```python
from build123d import *

# Parameters (mm, degrees)
SKETCH1_W           = 27.94
SKETCH1_H           = 391.16
BOSS_EXTRUDE1_DEPTH = 3.81
SKETCH2_R           = 10
CUT_EXTRUDE1_DEPTH  = 3.21
BOSS_EXTRUDE2_DEPTH = 3.81
SKETCH5_W           = 46.80460671
SKETCH5_H           = 4.064
CUT_EXTRUDE2_DEPTH  = 182.88
BOSS_EXTRUDE3_DEPTH = 3.81


with BuildPart() as part:
    # Sketch1 → Boss-Extrude1 (new body)
    with BuildSketch(Plane(origin=(0, 0, 0), x_dir=(1, 0, 0), z_dir=(0, 1, 0))):
        Rectangle(SKETCH1_W, SKETCH1_H)
    extrude(amount=BOSS_EXTRUDE1_DEPTH)

    # Sketch2 → Cut-Extrude1 (cut)
    with BuildSketch(Plane(origin=(0, 3.81, 0), x_dir=(1, 0, 0), z_dir=(0, 1, 0))):
        with Locations(Location((0, 177.8, 0), (0, 0, 270))):
            Circle(SKETCH2_R)
        with Locations(Location((0, 152.4, 0), (0, 0, 270))):
            Circle(SKETCH2_R)
        with Locations(Location((0, 127, 0), (0, 0, 270))):
            Circle(SKETCH2_R)
        with Locations(Location((0, 101.6, 0), (0, 0, 270))):
            Circle(SKETCH2_R)
        with Locations(Location((0, 76.2, 0), (0, 0, 270))):
            Circle(SKETCH2_R)
        with Locations(Location((0, 50.8, 0), (0, 0, 270))):
            Circle(SKETCH2_R)
        with Locations(Location((0, 25.4, 0), (0, 0, 270))):
            Circle(SKETCH2_R)
        with Locations(Location((0, 0, 0), (0, 0, 270))):
            Circle(SKETCH2_R)
        with Locations(Location((0, -25.4, 0), (0, 0, 270))):
            Circle(SKETCH2_R)
        with Locations(Location((0, -50.8, 0), (0, 0, 270))):
            Circle(SKETCH2_R)
        with Locations(Location((0, -76.2, 0), (0, 0, 270))):
            Circle(SKETCH2_R)
        with Locations(Location((0, -101.6, 0), (0, 0, 270))):
            Circle(SKETCH2_R)
        with Locations(Location((0, -127, 0), (0, 0, 270))):
            Circle(SKETCH2_R)
        with Locations(Location((0, -152.4, 0), (0, 0, 270))):
            Circle(SKETCH2_R)
        with Locations(Location((0, -177.8, 0), (0, 0, 270))):
            Circle(SKETCH2_R)
    extrude(amount=-CUT_EXTRUDE1_DEPTH, mode=Mode.SUBTRACT)

    # Sketch4 → Boss-Extrude2 (add)
    with BuildSketch(Plane(origin=(0, 0, 0), x_dir=(1, 0, 0), z_dir=(0, 1, 0))):
        Polygon((23.402303355, -54.881033493), (13.97, -56.20665728), (13.97, -72.402209707), (23.402303355, -73.727833493), align=None)
        Polygon((23.402303355, 146.105623787), (13.97, 144.78), (13.97, 128.584447573), (23.402303355, 127.258823787), align=None)
        Polygon((-13.97, 128.584447573), (-13.97, 144.78), (-23.402303355, 146.105623787), (-23.402303355, 127.258823787), align=None)
        Polygon((23.402303355, 79.11007136), (13.97, 77.784447573), (13.97, 61.588895147), (23.402303355, 60.26327136), align=None)
        Polygon((23.402303355, 12.114518933), (13.97, 10.788895147), (13.97, -5.40665728), (23.402303355, -6.732281067), align=None)
        Polygon((-13.97, -5.40665728), (-13.97, 10.788895147), (-23.402303355, 12.114518933), (-23.402303355, -6.732281067), align=None)
        Polygon((-13.97, 61.588895147), (-13.97, 77.784447573), (-23.402303355, 79.11007136), (-23.402303355, 60.26327136), align=None)
        Polygon((23.402303355, -121.87658592), (13.97, -123.202209707), (13.97, -139.397762134), (23.402303355, -140.72338592), align=None)
        Polygon((-13.97, -139.397762134), (-13.97, -123.202209707), (-23.402303355, -121.87658592), (-23.402303355, -140.72338592), align=None)
        Polygon((-13.97, -72.402209707), (-13.97, -56.20665728), (-23.402303355, -54.881033493), (-23.402303355, -73.727833493), align=None)
    extrude(amount=BOSS_EXTRUDE2_DEPTH)

    # Sketch5 → Cut-Extrude2 (cut)
    with BuildSketch(Plane.XY.offset(195.58)):
        with Locations((0, 2.032)):
            Rectangle(SKETCH5_W, SKETCH5_H)
    extrude(amount=-CUT_EXTRUDE2_DEPTH, mode=Mode.SUBTRACT)

    # Sketch6 → Boss-Extrude3 (add)
    with BuildSketch(Plane(origin=(0, 3.81, 0), x_dir=(1, 0, 0), z_dir=(0, 1, 0))):
        Polygon((-4.80197372, -12.7), (-4.445, -15.24), (-13.97, -15.24), (-13.97, -12.7), align=None)
        Polygon((13.97, -12.7), (13.97, -15.24), (4.445, -15.24), (4.80197372, -12.7), align=None)
    extrude(amount=-BOSS_EXTRUDE3_DEPTH)


solid = part.part
```
Could you check a few things on this model? Use its own coordinates, in mm. A direction names the side the tool comes from. Give positions to 0.01 mm unless a question says otherwise; leave off trailing zeros. Loops run counter-clockwise (first coordinate to the right, second up) from the corner with the lowest first, then second, coordinate; pieces in that order, holes last. Notation, with made-up numbers: (52.5, 58) - (79.5, 58) arc R9 cw to (79.5, 62) - close; hole circle Ø8 at (37.25, 61). An arc over 180 degrees is marked (long way). Answer in a Markdown table with one row per item. Add a question column.
Q1. If we section it at C-C (y = 1.45): State how many separate pieces and enclosed holes the cut face has, plus the area to 3 significant figures.
Q2. We'd pull the mould along Z, two halves only. Please class faces 4 (the face through (13.97, 2, 10)), 5 (the face through (-18.752, 1.878, -127.912)), 6 (the face through (18.62, 1.878, -60.935)), 7 (the face through (-18.62, 1.878, -145.434)): +Z half, -Z half, draft (parallel to the pull), parting line (faces both ways), or undercut.
Q3. If we section it at B-B (z = 0): List the corners of the cut face in (x, y) for me, plus the area to 3 significant figures.
Q4. If we section it at D-D (z = -101.6): List the corners of the cut face in (x, y) for me.
Q5. Please list where these lines run through material, in increasing order: L1, parallel to X at y = 1.05, z = -153; L2, parallel to Z at x = 19, y = 1.2; L3, parallel to Z at x = 21, y = 1.85. Write a range as from..to.
Q6. Which directions (+Z, -Z, +X, -X, +Y, -Y) give clear straight access to the entire face, cutting with the end or side of a thin tool? Please do faces 1 (the face through (18.62, 1.88, -127.93)), 2 (the face through (-23.402, 2, -137)), 3 (the face through (0, 0.6, -51)).
Q7. If we section it at A-A (x = -19): List the corners of the cut face in (y, z) for me, plus the area to 3 significant figures.
Q8. For pin 1 (2 mm diameter, centred on x = 7.5, z = -129, fed in from +Y); pin 2 (1.1 mm diameter, centred on y = 2, z = -109, fed in from -X); pin 3 (1.1 mm diameter, centred on x = 2, y = 2, fed in from +Z), each with a flat end and sliding along its axis, tell me the tip position at first contact or that it passes through.
The answers:
| question | item | result |
|---|---|---|
| 1 | separate pieces | 1 |
| 1 | enclosed holes | 8 |
| 1 | area | 4,350 mm^2 |
| 2 | face 4 | draft |
| 2 | face 5 | undercut |
| 2 | face 6 | undercut |
| 2 | face 7 | -Z half |
| 3 | outline | (-23.4, 0) - (23.4, 0) - (23.4, 3.81) - (10, 3.81) - (10, 0.6) - (-10, 0.6) - (-10, 3.81) - (-23.4, 3.81) - close |
| 3 | area | 114 mm^2 |
| 4 | outline | (-13.97, 0) - (13.97, 0) - (13.97, 3.81) - (10, 3.81) - (10, 0.6) - (-10, 0.6) - (-10, 3.81) - (-13.97, 3.81) - close |
| 5 | L1 | x = -13.97..-9.98, 9.98..13.97 |
| 5 | L2 | z = -145.49..-127.88, -78.49..-60.88, -11.5..6.11 |
| 5 | L3 | z = -145.77..-127.6, -78.77..-60.6, -11.78..6.39 |
| 6 | face 1 | +Y, -Y |
| 6 | face 2 | +Z, -Z, -X, +Y, -Y |
| 6 | face 3 | +Y |
| 7 | outline | (0, -145.49) - (3.81, -145.49) - (3.81, -127.88) - (0, -127.88) - close; (0, -78.49) - (3.81, -78.49) - (3.81, -60.88) - (0, -60.88) - close; (0, -11.5) - (3.81, -11.5) - (3.81, 6.11) - (0, 6.11) - close |
| 7 | area | 201 mm^2 |
| 8 | pin 1 | stops at y = 0.6 |
| 8 | pin 2 | stops at x = -13.97 |
| 8 | pin 3 | stops at z = 12.7 |
